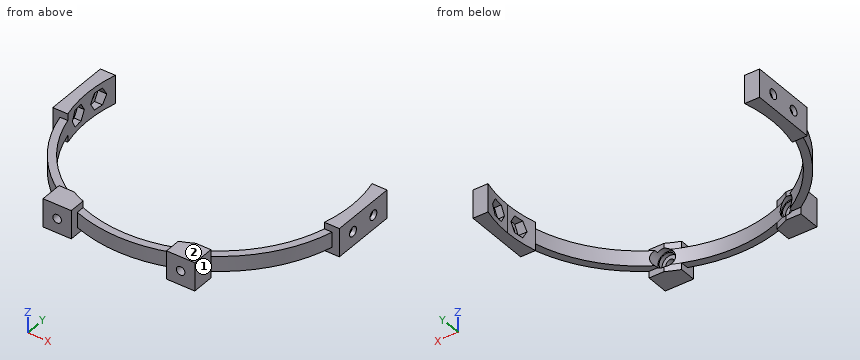
from build123d import *

# Parameters (mm, degrees)
BOSS_EXTRUDE1_DEPTH                            = 4
BOSS_EXTRUDE2_DEPTH                            = 7.5
CUT_EXTRUDE1_DEPTH                             = 3.5
F_8_0_199_DIAMETER_HOLE1_AT_2_COUNT            = 2
F_8_0_199_DIAMETER_HOLE1_AT_2_PITCH            = 15
BOSS_EXTRUDE3_REACH                            = 108.518
BOSS_EXTRUDE3_DIRECTION_2_REACH                = 108.518
SKETCH6_R                                      = 5
CUT_EXTRUDE2_DEPTH                             = 3.5
CUT_EXTRUDE2_DEPTH_BACK                        = 3
CBORE_FOR_8_BUTTON_HEAD_CAP_SCREW1_D           = 4.4958
CBORE_FOR_8_BUTTON_HEAD_CAP_SCREW1_DEPTH       = 11.649325414
CBORE_FOR_8_BUTTON_HEAD_CAP_SCREW1_CBORE_D     = 8.73252
CBORE_FOR_8_BUTTON_HEAD_CAP_SCREW1_CBORE_DEPTH = 2.2098
CBORE_FOR_8_BUTTON_HEAD_CAP_SCREW1_TIP         = 1.350674586


with BuildPart() as part:
    # Sketch1 → Boss-Extrude1 (new, symmetric)
    with BuildSketch(Plane.XY):
        with BuildLine():
            Line((-76, 17.5), (-76, 0))
            Line((-76, 0), (-76, -17.5))
            Line((-76, -17.5), (-72.163391169, -17.5))
            Line((-72.163391169, -17.5), (-68.04053957, -17.5))
            ThreePointArc((-68.04053957, -17.5), (-69.699186267, -8.81977657), (-70.255, 0))
            ThreePointArc((-70.255, 0), (-69.699186267, 8.81977657), (-68.04053957, 17.5))
            Line((-68.04053957, 17.5), (-70.255, 17.5))
            Line((-70.255, 17.5), (-76, 17.5))
        make_face()
        with BuildLine():
            Line((-68.04053957, -17.5), (-72.163391169, -17.5))
            ThreePointArc((-72.163391169, -17.5), (0, -74.255), (72.163391169, -17.5))
            Line((72.163391169, -17.5), (68.04053957, -17.5))
            ThreePointArc((68.04053957, -17.5), (0, -70.255), (-68.04053957, -17.5))
        make_face()
        with BuildLine():
            Line((68.04053957, -17.5), (72.163391169, -17.5))
            Line((72.163391169, -17.5), (76, -17.5))
            Line((76, -17.5), (76, 0))
            Line((76, 0), (76, 17.5))
            Line((76, 17.5), (70.255, 17.5))
            Line((70.255, 17.5), (68.04053957, 17.5))
            ThreePointArc((68.04053957, 17.5), (69.699186267, 8.81977657), (70.255, 0))
            ThreePointArc((70.255, 0), (69.699186267, -8.81977657), (68.04053957, -17.5))
        make_face()
    extrude(amount=BOSS_EXTRUDE1_DEPTH, both=True)

    # Sketch1<5> → Boss-Extrude2 (add, symmetric)
    with BuildSketch(Plane.XY):
        with BuildLine():
            Line((-76, 17.5), (-76, 0))
            Line((-76, 0), (-76, -17.5))
            Line((-76, -17.5), (-72.163391169, -17.5))
            Line((-72.163391169, -17.5), (-68.04053957, -17.5))
            ThreePointArc((-68.04053957, -17.5), (-69.699186267, -8.81977657), (-70.255, 0))
            ThreePointArc((-70.255, 0), (-69.699186267, 8.81977657), (-68.04053957, 17.5))
            Line((-68.04053957, 17.5), (-70.255, 17.5))
            Line((-70.255, 17.5), (-76, 17.5))
        make_face()
        with BuildLine():
            Line((68.04053957, -17.5), (72.163391169, -17.5))
            Line((72.163391169, -17.5), (76, -17.5))
            Line((76, -17.5), (76, 0))
            Line((76, 0), (76, 17.5))
            Line((76, 17.5), (70.255, 17.5))
            Line((70.255, 17.5), (68.04053957, 17.5))
            ThreePointArc((68.04053957, 17.5), (69.699186267, 8.81977657), (70.255, 0))
            ThreePointArc((70.255, 0), (69.699186267, -8.81977657), (68.04053957, -17.5))
        make_face()
    extrude(amount=BOSS_EXTRUDE2_DEPTH, both=True)

    # Sketch2 → Cut-Extrude1 (cut, symmetric)
    with BuildSketch(Plane.ZY.offset(-70.255)):
        Polygon((0, 2.332715091), (4.475, 4.916357545), (4.475, 10.083642455), (0, 12.667284909), (-4.475, 10.083642455), (-4.475, 4.916357545), align=None)
        Polygon((0, -12.667284909), (4.475, -10.083642455), (4.475, -4.916357545), (0, -2.332715091), (-4.475, -4.916357545), (-4.475, -10.083642455), align=None)
    cut_extrude1 = extrude(amount=CUT_EXTRUDE1_DEPTH, both=True, mode=Mode.SUBTRACT)

    # Sketch4 → #8 (0.199) Diameter Hole1 (revolve, cut)
    with BuildSketch(Plane(origin=(76, 7.5, 0), x_dir=(0, 0, -1), z_dir=(0, 1, 0))):
        Polygon((0, 0), (0, 10.71), (2.5273, 9.191444958), (2.5273, 0), align=None)
    f_8_0_199_diameter_hole1 = revolve(axis=Axis((82.35, 7.5, 0), (-1, 0, 0)), mode=Mode.SUBTRACT)

    # #8 (0.199) Diameter Hole1 at 2: #8 (0.199) Diameter Hole1 ×2
    with Locations(*[(0, -i * F_8_0_199_DIAMETER_HOLE1_AT_2_PITCH, 0) for i in range(1, F_8_0_199_DIAMETER_HOLE1_AT_2_COUNT)]):
        add(f_8_0_199_diameter_hole1, mode=Mode.SUBTRACT)

    # Mirror1: Cut-Extrude1, #8 (0.199) Diameter Hole1 across plane
    add(cut_extrude1.mirror(Plane(origin=(0, 0, 0), x_dir=(0, 0, 1), z_dir=(1, 0, 0))), mode=Mode.SUBTRACT)
    add(f_8_0_199_diameter_hole1.mirror(Plane(origin=(0, 0, 0), x_dir=(0, 0, 1), z_dir=(1, 0, 0))), mode=Mode.SUBTRACT)

    # Mirror1 copy 1 sketch → Mirror1 copy 1 (revolve, cut)
    with BuildSketch(Plane(origin=(-76, -7.5, 0), x_dir=(0, 0, -1), z_dir=(0, 1, 0))):
        Polygon((0, 0), (0, -10.71), (2.5273, -9.191444958), (2.5273, 0), align=None)
    revolve(axis=Axis((-82.35, -7.5, 0), (-1, 0, 0)), mode=Mode.SUBTRACT)

    # Boss-Extrude3: up to this face of the body (flat: up to its plane)
    boss_extrude3_end = Plane(part.part.faces().sort_by_distance((-72.727295349, 0, 7.5))[0])
    # Sketch5 → Boss-Extrude3 (add, up to the picked face)
    with BuildSketch(Plane.XY, mode=Mode.PRIVATE) as boss_extrude3_sk1:
        with BuildLine():
            Line((40.25, -62.399859976), (40.25, -74.255))
            Line((40.25, -74.255), (25.25, -74.255))
            Line((25.25, -74.255), (25.25, -65.560678192))
            ThreePointArc((25.25, -65.560678192), (28.808569138, -64.076761538), (32.280373294, -62.399859976))
            Line((32.280373294, -62.399859976), (40.25, -62.399859976))
        make_face()
    boss_extrude3_tool1 = split(extrude(boss_extrude3_sk1.sketch, amount=BOSS_EXTRUDE3_REACH, mode=Mode.PRIVATE), bisect_by=boss_extrude3_end, keep=Keep.BOTH, mode=Mode.PRIVATE)
    # Sketch5 → Boss-Extrude3 (add, up to the picked face)
    with BuildSketch(Plane.XY, mode=Mode.PRIVATE) as boss_extrude3_sk2:
        with BuildLine():
            Line((-25.25, -74.255), (-40.25, -74.255))
            Line((-40.25, -74.255), (-40.25, -62.399859976))
            Line((-40.25, -62.399859976), (-32.280373294, -62.399859976))
            ThreePointArc((-32.280373294, -62.399859976), (-28.808569138, -64.076761538), (-25.25, -65.560678192))
            Line((-25.25, -65.560678192), (-25.25, -74.255))
        make_face()
    boss_extrude3_tool2 = split(extrude(boss_extrude3_sk2.sketch, amount=BOSS_EXTRUDE3_REACH, mode=Mode.PRIVATE), bisect_by=boss_extrude3_end, keep=Keep.BOTH, mode=Mode.PRIVATE)
    add(boss_extrude3_tool1.solids().sort_by(Axis((33.107767, -68.667419, 0), (0, 0, 1)))[0])
    add(boss_extrude3_tool2.solids().sort_by(Axis((-33.107767, -68.667419, 0), (0, 0, 1)))[0])

    # Boss-Extrude3 direction 2: up to this face of the body (flat: up to its plane)
    boss_extrude3_direction_2_end = Plane(part.part.faces().sort_by_distance((-72.727295349, 0, -7.5))[0])
    # Sketch5 → Boss-Extrude3 direction 2 (add, up to the picked face)
    with BuildSketch(Plane.XY, mode=Mode.PRIVATE) as boss_extrude3_direction_2_sk1:
        with BuildLine():
            Line((40.25, -62.399859976), (40.25, -74.255))
            Line((40.25, -74.255), (25.25, -74.255))
            Line((25.25, -74.255), (25.25, -65.560678192))
            ThreePointArc((25.25, -65.560678192), (28.808569138, -64.076761538), (32.280373294, -62.399859976))
            Line((32.280373294, -62.399859976), (40.25, -62.399859976))
        make_face()
    boss_extrude3_direction_2_tool1 = split(extrude(boss_extrude3_direction_2_sk1.sketch, amount=-BOSS_EXTRUDE3_DIRECTION_2_REACH, mode=Mode.PRIVATE), bisect_by=boss_extrude3_direction_2_end, keep=Keep.BOTH, mode=Mode.PRIVATE)
    # Sketch5 → Boss-Extrude3 direction 2 (add, up to the picked face)
    with BuildSketch(Plane.XY, mode=Mode.PRIVATE) as boss_extrude3_direction_2_sk2:
        with BuildLine():
            Line((-25.25, -74.255), (-40.25, -74.255))
            Line((-40.25, -74.255), (-40.25, -62.399859976))
            Line((-40.25, -62.399859976), (-32.280373294, -62.399859976))
            ThreePointArc((-32.280373294, -62.399859976), (-28.808569138, -64.076761538), (-25.25, -65.560678192))
            Line((-25.25, -65.560678192), (-25.25, -74.255))
        make_face()
    boss_extrude3_direction_2_tool2 = split(extrude(boss_extrude3_direction_2_sk2.sketch, amount=-BOSS_EXTRUDE3_DIRECTION_2_REACH, mode=Mode.PRIVATE), bisect_by=boss_extrude3_direction_2_end, keep=Keep.BOTH, mode=Mode.PRIVATE)
    add(boss_extrude3_direction_2_tool1.solids().sort_by(Axis((33.107767, -68.667419, 0), (0, 0, -1)))[0])
    add(boss_extrude3_direction_2_tool2.solids().sort_by(Axis((-33.107767, -68.667419, 0), (0, 0, -1)))[0])

    # Sketch6 → Cut-Extrude2 (cut, two sides)
    with BuildSketch(Plane(origin=(0, -62.399859976, 0), x_dir=(1, 0, 0), z_dir=(0, 1, 0))) as cut_extrude2_sk:
        with Locations(Location((-32.75, 0, 0), (0, 0, 84.610530172))):
            Circle(SKETCH6_R)
        with Locations(Location((32.75, 0, 0), (0, 0, 95.389469991))):
            Circle(SKETCH6_R)
    extrude(amount=CUT_EXTRUDE2_DEPTH, mode=Mode.SUBTRACT)
    extrude(cut_extrude2_sk.sketch, amount=-CUT_EXTRUDE2_DEPTH_BACK, mode=Mode.SUBTRACT)

    # CBORE for #8 Button Head Cap Screw1
    with Locations(Plane(origin=(-32.75, -65.399859976, 0), x_dir=(0, 0, 1), z_dir=(0, 1, 0))):
        with Locations((0, 0), (0, 65.5)):
            CounterBoreHole(CBORE_FOR_8_BUTTON_HEAD_CAP_SCREW1_D / 2, CBORE_FOR_8_BUTTON_HEAD_CAP_SCREW1_CBORE_D / 2, CBORE_FOR_8_BUTTON_HEAD_CAP_SCREW1_CBORE_DEPTH, depth=CBORE_FOR_8_BUTTON_HEAD_CAP_SCREW1_DEPTH)
            with Locations((0, 0, -(CBORE_FOR_8_BUTTON_HEAD_CAP_SCREW1_DEPTH + CBORE_FOR_8_BUTTON_HEAD_CAP_SCREW1_TIP / 2))):  # 118° drill point
                Cone(0, CBORE_FOR_8_BUTTON_HEAD_CAP_SCREW1_D / 2, CBORE_FOR_8_BUTTON_HEAD_CAP_SCREW1_TIP, mode=Mode.SUBTRACT)


solid = part.part
Could you check a few things on this model? Use its own coordinates, in mm. Face numbers are marked on the shaded views. A direction names the side the tool comes from. Give positions to 0.01 mm unless a question says otherwise; leave off trailing zeros. Write each loop counter-clockwise with the first axis right and the second up, starting at its lowest first coordinate (ties: lowest second). Pieces come first, ordered by that corner, then holes. Notation, with made-up numbers: (73, -30.75) -> (86, -30.75) arc R26 cw to (86, -7.75) -> close; hole circle Ø10 at (7, -5). An arc over 180 degrees is marked (long way). Answer as CSV lines item,"result". Start each with the question number.
(1) If we section it at B-B, the plane y = -38: Write out the boundary of the cut face in (x, z), and give its area (3 significant figures).
(2) Please list where these lines run through material, in increasing order: line 1 (Y direction, x = 74.85, z = 0); line 2 (Z direction, x = -75.25, y = -7.5); line 3 (X direction, y = -55, z = -3).
(3) If we section it at D-D, the plane x = 5: Write out the boundary of the cut face in (y, z), and give its area (3 significant figures).
(4) I'm going to push flat-ended pins straight in: pin 1 Ø1.5 at (x, z) = (49, 0.5) entering from +Y; pin 2 Ø7 at (x, y) = (2.5, -70) entering from +Z; pin 3 Ø1 at (x, z) = (9, -3) entering from -Y. Where does each tip first touch, or does it pass through?
(5) If we section it at A-A, the plane y = 7.5: Write out the boundary of the cut face in (x, z) (3 decimals).
(6) If we section it at C-C, the plane x = -54: Write out the boundary of the cut face in (y, z).
(7) Which directions (+Z, -Z, +X, -X, +Y, -Y) give clear straight access to the entire face, cutting with the end or side of a thin tool? Please do the marked faces 1 and 2.
Answer list:
1,outline,"(-63.8, -4) -> (-59.09, -4) -> (-59.09, 4) -> (-63.8, 4) -> close; (59.09, -4) -> (63.8, -4) -> (63.8, 4) -> (59.09, 4) -> close"
1,area,"75.3 mm^2"
2,line 1,"-17.5 to -10.03, -4.97 to 4.97, 10.03 to 17.5"
2,line 2,"-7.5 to -2.53, 2.53 to 7.5"
2,line 3,"-49.89 to -43.71, 43.71 to 49.89"
3,outline,"(-74.09, -4) -> (-70.08, -4) -> (-70.08, 4) -> (-74.09, 4) -> close"
3,area,"32.1 mm^2"
4,pin 1,"y = -49.61"
4,pin 2,"z = 4"
4,pin 3,"y = -73.77"
5,outline,"(-76, -7.5) -> (-69.854, -7.5) -> (-69.854, -4.475) -> (-73.755, -4.475) -> (-73.755, -2.527) -> (-76, -2.527) -> close; (-76, 2.527) -> (-73.755, 2.527) -> (-73.755, 4.475) -> (-69.854, 4.475) -> (-69.854, 7.5) -> (-76, 7.5) -> close; (69.854, -7.5) -> (76, -7.5) -> (76, -2.527) -> (73.755, -2.527) -> (73.755, -4.475) -> (69.854, -4.475) -> close; (69.854, 4.475) -> (73.755, 4.475) -> (73.755, 2.527) -> (76, 2.527) -> (76, 7.5) -> (69.854, 7.5) -> close"
6,outline,"(-50.97, -4) -> (-44.94, -4) -> (-44.94, 4) -> (-50.97, 4) -> close"
7,face 1,"+Z, -Z, +X, -Y"
7,face 2,"+Z, +X, -X, +Y, -Y"
